Design review of the part built by this model. Coordinates are the model's own, in mm. Give positions to 0.01 mm unless a question says otherwise; leave off trailing zeros. Loops run counter-clockwise (first coordinate to the right, second up) from the corner with the lowest first, then second, coordinate; pieces in that order, holes last.
from build123d import *

# Parameters (mm, degrees)
F0_R     = 2
F0_R_2   = 60
F1_DEPTH = 25


with BuildPart() as f1:
    # F0 (on Top) → F1 (new body)
    with BuildSketch(Plane.XY):
        with BuildLine():
            Line((70, 75), (-70, 75))
            ThreePointArc((-70, 75), (-73.535534, 73.535534), (-75, 70))
            Line((-75, 70), (-75, -70))
            ThreePointArc((-75, -70), (-73.535534, -73.535534), (-70, -75))
            Line((-70, -75), (70, -75))
            ThreePointArc((70, -75), (73.535534, -73.535534), (75, -70))
            Line((75, -70), (75, 70))
            ThreePointArc((75, 70), (73.535534, 73.535534), (70, 75))
        make_face()
        with Locations((-52.4, -52.4)):
            Circle(F0_R, mode=Mode.SUBTRACT)
        with Locations((52.4, -52.4)):
            Circle(F0_R, mode=Mode.SUBTRACT)
        with Locations((-52.4, 52.4)):
            Circle(F0_R, mode=Mode.SUBTRACT)
        Circle(F0_R_2, mode=Mode.SUBTRACT)
        with Locations((52.4, 52.4)):
            Circle(F0_R, mode=Mode.SUBTRACT)
    extrude(amount=F1_DEPTH)


solid = f1.part
Q1. Take a section at D-D (x = 52.4). Give the boundary of the cut face in (y, z).
Results:
outline: (-75, 0) - (-54.4, 0) - (-54.4, 25) - (-75, 25) - close; (-50.4, 0) - (-29.23, 0) - (-29.23, 25) - (-50.4, 25) - close; (29.23, 0) - (50.4, 0) - (50.4, 25) - (29.23, 25) - close; (54.4, 0) - (75, 0) - (75, 25) - (54.4, 25) - close
Q2. Draft analysis for pull direction Y (two halves, no side actions). For faces 1 (the face through (-1, -75, 12)), 2 (the face through (-75, 1, 12)), 3 (the face through (53.323, 50.626, 12.325)), state which applies: pulls with the +Y half, pulls with the -Y half, needs draft (parallel to the pull), parting line crosses it, or undercut.
Results:
face 1: pulls with the -Y half
face 2: needs draft
face 3: undercut
Q3. Take a section at C-C (z = 9.25). Give the boundary of the cut face in (x, y), plus the area to 3 significant figures.
Results:
outline: (-75, -70) arc R5 ccw to (-70, -75) - (70, -75) arc R5 ccw to (75, -70) - (75, 70) arc R5 ccw to (70, 75) - (-70, 75) arc R5 ccw to (-75, 70) - close; hole circle Ø120 at (0, 0); hole circle Ø4 at (-52.4, -52.4); hole circle Ø4 at (-52.4, 52.4); hole circle Ø4 at (52.4, -52.4); hole circle Ø4 at (52.4, 52.4)
area: 11,100 mm2
Q4. Take a section at B-B (x = -24). Give the boundary of the cut face in (y, z).
Results:
outline: (-75, 0) - (-54.99, 0) - (-54.99, 25) - (-75, 25) - close; (54.99, 0) - (75, 0) - (75, 25) - (54.99, 25) - close
Q5. Wall thickness on line 1 (Y direction, x = -52.4, z = 15.75); line 2 (Y direction, x = 0, z = 6.75); line 3 (Y direction, x = -32.5, z = 17.5): over which ranges is each line inside the solid? List them lowest first.
Results:
line 1: y = -75 to -54.4, -50.4 to -29.23, 29.23 to 50.4, 54.4 to 75
line 2: y = -75 to -60, 60 to 75
line 3: y = -75 to -50.44, 50.44 to 75
Q6. Insertion check: pin 1 (3 mm diameter, centred on x = -52.4, y = -52.4, fed in from +Z). The pin has a flat end and moves straight along its axis. Give the tip position at first contact, or say it passes through.
Results:
pin 1: passes through
Q7. Take a section at A-A (y = 0). Give the boundary of the cut face in (x, z).
Results:
outline: (-75, 0) - (-60, 0) - (-60, 25) - (-75, 25) - close; (60, 0) - (75, 0) - (75, 25) - (60, 25) - close
